from build123d import *

# Parameters (mm, degrees)
SKETCH1_W           = 25
SKETCH1_H           = 25
BOSS_EXTRUDE1_DEPTH = 28
SKETCH2_R           = 5
CUT_EXTRUDE1_DEPTH  = 30
SKETCH3_R           = 7.5
CUT_EXTRUDE2_DEPTH  = 25
BOSS_EXTRUDE2_DEPTH = 28
FILLET1_R           = 5
SKETCH7_R           = 1.75
CUT_EXTRUDE3_DEPTH  = 13
SKETCH8_R           = 3
CUT_EXTRUDE4_DEPTH  = 18


with BuildPart() as part:
    # Sketch1 → Boss-Extrude1 (new body)
    with BuildSketch(Plane(origin=(0, 0, 0), x_dir=(1, 0, 0), z_dir=(0, 1, 0))):
        Rectangle(SKETCH1_W, SKETCH1_H)
    extrude(amount=BOSS_EXTRUDE1_DEPTH)

    # Sketch2 → Cut-Extrude1 (cut)
    with BuildSketch(Plane(origin=(0, 28, 0), x_dir=(1, 0, 0), z_dir=(0, 1, 0))):
        with Locations(Location((0, 0, 0), (0, 0, 270))):
            Circle(SKETCH2_R)
    extrude(amount=-CUT_EXTRUDE1_DEPTH, mode=Mode.SUBTRACT)

    # Sketch3 → Cut-Extrude2 (cut)
    with BuildSketch(Plane(origin=(0, 28, 0), x_dir=(1, 0, 0), z_dir=(0, 1, 0))):
        with Locations(Location((0, 0, 0), (0, 0, 270))):
            Circle(SKETCH3_R)
    extrude(amount=-CUT_EXTRUDE2_DEPTH, mode=Mode.SUBTRACT)

    # Sketch6 → Boss-Extrude2 (add)
    with BuildSketch(Plane.XZ):
        Polygon((-12.5, -12.5), (-12.5, -27.5), (-7.5, -27.5), (0, -12.5), align=None)
        Polygon((-7.5, 27.5), (0, 12.5), (-12.5, 12.5), (-12.5, 27.5), align=None)
    extrude(amount=-BOSS_EXTRUDE2_DEPTH)

    # Fillet1
    fillet1_edges = [part.edges().sort_by_distance(p)[0] for p in [
        (0, 14, -12.5),
        (0, 14, 12.5),
    ]]
    fillet(fillet1_edges, radius=FILLET1_R)

    # Sketch7 → Cut-Extrude3 (cut)
    with BuildSketch(Plane.ZY.offset(12.5)):
        with Locations((20, 20)):
            Circle(SKETCH7_R)
        with Locations((20, 5)):
            Circle(SKETCH7_R)
        with Locations(Location((-20, 20, 0), (0, 0, 180))):
            Circle(SKETCH7_R)
        with Locations(Location((-20, 5, 0), (0, 0, 180))):
            Circle(SKETCH7_R)
    extrude(amount=-CUT_EXTRUDE3_DEPTH, mode=Mode.SUBTRACT)

    # Sketch8 → Cut-Extrude4 (cut)
    with BuildSketch(Plane(origin=(12.5, 0, 0), x_dir=(0, 0, -1), z_dir=(1, 0, 0))):
        with Locations((20, 20)):
            Circle(SKETCH8_R)
        with Locations((20, 5)):
            Circle(SKETCH8_R)
        with Locations((-20, 20)):
            Circle(SKETCH8_R)
        with Locations((-20, 5)):
            Circle(SKETCH8_R)
    extrude(amount=-CUT_EXTRUDE4_DEPTH, mode=Mode.SUBTRACT)


solid = part.part
Work out the finished part from the listing and answer in its coordinate system (mm). A direction names the side the tool comes from. Round coordinates to 2 decimals unless told otherwise and drop trailing zeros. Order: outer loops, then holes, each group sorted by start corner. A loop starts at its lowest first (then second) coordinate and runs counter-clockwise, first axis right, second up. Notation, with made-up numbers: M 86.5,-16 L 134.5,-16 A25 ccw 134.5,10 Z; hole C 64,40 d3. An arc over 180 degrees is marked long. One line per item, written item: value.
Q1. Flat-ended cylindrical pins translate along their axes: pin 1 (6.5 mm diameter, centred on y = 19, z = -20, fed in from +X) (3 decimals); pin 2 (12 mm diameter, centred on x = 6.5, y = 14, fed in from +Z); pin 3 (5 mm diameter, centred on x = 2, y = 18.5, fed in from -Z). Find the tip coordinate at first contact, or state that the pin passes through.
Derived:
pin 1: x = -2.125
pin 2: z = 13.22
pin 3: z = -14.02
Q2. Find section C-C on x = -9.5. Write down the section's boundary in (y, z), then the cut area to 3 significant figures.
Derived:
outline: M 0,-27.5 L 28,-27.5 L 28,27.5 L 0,27.5 Z; hole C 5,-20 d3.5; hole C 5,20 d3.5; hole C 20,-20 d3.5; hole C 20,20 d3.5
area: 1,500 mm²
Q3. Find section D-D on x = 0. Write down the section's boundary in (y, z), then the cut area to 3 significant figures.
Derived:
outline: M 0,-13.57 L 28,-13.57 L 28,-7.5 L 3,-7.5 L 3,-5 L 0,-5 Z; M 0,5 L 3,5 L 3,7.5 L 28,7.5 L 28,13.57 L 0,13.57 Z
area: 355 mm²
Q4. Straight lines are drawn through the part: line 1 (Y direction, x = -6.75, z = 20); line 2 (X direction, y = 1.7, z = 0); line 3 (Z direction, x = 4.75, y = 16.75). For each, find the intervals that lie inside material, in ascending order.
Derived:
line 1: 0 to 3.25, 6.75 to 18.25, 21.75 to 28
line 2: -12.5 to -5, 5 to 12.5
line 3: -12.5 to -5.8, 5.8 to 12.5
Q5. For faces 5 (the face through (0.33, 15.675, -7.493)), 6 (the face through (-4, 20, -17)), 7 (the face through (-9.05, 21.18, 18.71)), determine the directions among +Z, -Z, +X, -X, +Y, -Y from which every point of the face is accessible in a straight line to the end or side of a thin tool.
Derived:
face 5: +Y
face 6: +X
face 7: +X, -X
Q6. Determine the mould class of faces 1 (the face through (8, 14, -12.5)), 2 (the face through (-4.5, 13.8, 21.5)), 3 (the face through (-5, 3, 2)), 4 (the face through (-5.5, 5, 18)) for opening direction Z: released by +Z, released by -Z, zero draft, split by the parting line, or undercut.
Derived:
face 1: released by -Z
face 2: released by +Z
face 3: undercut
face 4: undercut
Q7. Find section B-B on z = 20. Write down the section's boundary in (x, y), then the cut area to 3 significant figures.
Derived:
outline: M -12.5,0 L -3.75,0 L -3.75,2 L -5.5,2 L -5.5,3.25 L -12.5,3.25 Z; M -12.5,6.75 L -5.5,6.75 L -5.5,8 L -3.75,8 L -3.75,17 L -5.5,17 L -5.5,18.25 L -12.5,18.25 Z; M -12.5,21.75 L -5.5,21.75 L -5.5,23 L -3.75,23 L -3.75,28 L -12.5,28 Z
area: 175 mm²
Q8. Find section A-A on y = 5. Write down the section's boundary in (x, z), then the cut area to 3 significant figures.
Derived:
outline: M -12.5,-27.5 L -7.5,-27.5 L -5.25,-23 L -5.5,-23 L -5.5,-21.75 L -12.5,-21.75 Z; M -12.5,-18.25 L -5.5,-18.25 L -5.5,-17 L -2.25,-17 L -1.38,-15.26 A5 cw 3.09,-12.5 L 12.5,-12.5 L 12.5,12.5 L 3.09,12.5 A5 cw -1.38,15.26 L -2.25,17 L -5.5,17 L -5.5,18.25 L -12.5,18.25 Z; M -12.5,21.75 L -5.5,21.75 L -5.5,23 L -5.25,23 L -7.5,27.5 L -12.5,27.5 Z; hole C 0,0 d15
area: 644 mm²
